The model under review builds one solid part; all positions refer to its coordinate system, in mm. A direction names the side the tool comes from. Coordinates: 2 decimals unless noted, no trailing zeros. Order: outer loops, then holes, each group sorted by start corner. A loop starts at its lowest first (then second) coordinate and runs counter-clockwise, first axis right, second up. Notation, with made-up numbers: M 34,42 L 80,42 A16 ccw 80,71 Z; hole C 23,-19.75 d2. An arc over 180 degrees is marked long. Write each question's results on one line, items separated by ' | '.
from build123d import *

# Parameters (mm, degrees)
SKETCH1_W                    = 168.275
SKETCH1_H                    = 76.2
EXTRUDE1_DEPTH               = 57.15
SKETCH2_R                    = 12.7
EXTRUDE2_DEPTH               = 6.35
SKETCH3_R                    = 9.525
EXTRUDE3_DEPTH               = 38.1
F_5_16_18_TAPPED_HOLE1_D     = 6.5278
F_5_16_18_TAPPED_HOLE1_DEPTH = 22.9235
F_5_16_18_TAPPED_HOLE1_TIP   = 1.961148974
SKETCH7_R                    = 36.83
EXTRUDE4_DEPTH               = 68.072
SKETCH8_R                    = 38.481
EXTRUDE5_DEPTH               = 25.4
F_5_16_18_TAPPED_HOLE2_D     = 6.5278
F_5_16_18_TAPPED_HOLE2_DEPTH = 22.922992
F_5_16_18_TAPPED_HOLE2_TIP   = 1.961148974
SKETCH11_OUTSIDE_W           = 224.478
SKETCH11_OUTSIDE_H           = 132.784
CUT_EXTRUDE1_DEPTH           = 9.525


with BuildPart() as part:
    # Sketch1 → Extrude1 (new body)
    with BuildSketch(Plane.XY):
        with Locations((41.7703, 0)):
            Rectangle(SKETCH1_W, SKETCH1_H)
    extrude(amount=-EXTRUDE1_DEPTH)

    # Sketch2 → Extrude2 (add)
    with BuildSketch(Plane.XY):
        Circle(SKETCH2_R)
    extrude(amount=EXTRUDE2_DEPTH)

    # Sketch3 → Extrude3 (add)
    with BuildSketch(Plane.XY.offset(6.35)):
        Circle(SKETCH3_R)
    extrude(amount=EXTRUDE3_DEPTH)

    # 5/16-18 Tapped Hole1
    with Locations(Plane.XZ.offset(38.1)):
        with Locations((-34.4297, -23.8125), (-34.4297, -49.2125), (117.9703, -49.2125), (117.9703, -23.8125)):
            Hole(F_5_16_18_TAPPED_HOLE1_D / 2, depth=F_5_16_18_TAPPED_HOLE1_DEPTH)
            with Locations((0, 0, -(F_5_16_18_TAPPED_HOLE1_DEPTH + F_5_16_18_TAPPED_HOLE1_TIP / 2))):  # 118° drill point
                Cone(0, F_5_16_18_TAPPED_HOLE1_D / 2, F_5_16_18_TAPPED_HOLE1_TIP, mode=Mode.SUBTRACT)

    # Sketch7 → Extrude4 (add)
    with BuildSketch(Plane(origin=(0, 0, -57.15), x_dir=(-1, 0, 0), z_dir=(0, 0, -1))):
        with Locations((-87.8078, 0)):
            Circle(SKETCH7_R)
    extrude(amount=EXTRUDE4_DEPTH)

    # Sketch8 → Extrude5 (add)
    with BuildSketch(Plane(origin=(0, 0, -125.222), x_dir=(-1, 0, 0), z_dir=(0, 0, -1))):
        with Locations((-87.8078, 0)):
            Circle(SKETCH8_R)
    extrude(amount=EXTRUDE5_DEPTH)

    # 5/16-18 Tapped Hole2
    with Locations(Plane(origin=(0, 38.1, 0), x_dir=(-1, 0, 0), z_dir=(0, 1, 0))):
        with Locations((34.4297, -23.8125), (34.4297, -49.2125), (-117.9703, -49.2125), (-117.9703, -23.8125)):
            Hole(F_5_16_18_TAPPED_HOLE2_D / 2, depth=F_5_16_18_TAPPED_HOLE2_DEPTH)
            with Locations((0, 0, -(F_5_16_18_TAPPED_HOLE2_DEPTH + F_5_16_18_TAPPED_HOLE2_TIP / 2))):  # 118° drill point
                Cone(0, F_5_16_18_TAPPED_HOLE2_D / 2, F_5_16_18_TAPPED_HOLE2_TIP, mode=Mode.SUBTRACT)

    # Sketch11 outside → Cut-Extrude1 (cut)
    with BuildSketch(Plane.XY):
        with Locations((41.961, 0)):
            Rectangle(SKETCH11_OUTSIDE_W, SKETCH11_OUTSIDE_H)
        with BuildLine():
            Line((89.393090644, 18.410189037), (27.411408932, 18.410189037))
            ThreePointArc((27.411408932, 18.410189037), (-33.006603821, 0.940480831), (26.318636507, -19.941157749))
            Line((26.318636507, -19.941157749), (89.393090644, -19.941157749))
            ThreePointArc((89.393090644, -19.941157749), (108.568764037, -0.765484356), (89.393090644, 18.410189037))
        make_face(mode=Mode.SUBTRACT)
    extrude(amount=-CUT_EXTRUDE1_DEPTH, mode=Mode.SUBTRACT)


solid = part.part
1) For pin 1 (8 mm diameter, centred on y = -9.5, z = -21.5, fed in from +X); pin 2 (8.5 mm diameter, centred on x = 117.97, z = -49.21, fed in from +Y); pin 3 (7.5 mm diameter, centred on x = 62.5, z = -3, fed in from +Y), all flat-tipped, find the tip position at first contact; note any pin that passes through.
Solutions:
pin 1: x = 125.91 | pin 2: y = 38.1 | pin 3: y = 18.41
2) Take a section at A-A on x = 0. State the section outline as (y, z) points (3 decimals), plus the area to 3 significant figures.
Solutions:
outline: M -38.1,-57.15 L 38.1,-57.15 L 38.1,-9.525 L 33.02,-9.525 L 33.02,0 L 12.7,0 L 12.7,6.35 L 9.525,6.35 L 9.525,44.45 L -9.525,44.45 L -9.525,6.35 L -12.7,6.35 L -12.7,0 L -33.02,0 L -33.02,-9.525 L -38.1,-9.525 Z | area: 5,150 mm2
3) Take a section at C-C on y = 0. State the section outline as (x, z) points (3 decimals), plus the area to 3 significant figures.
Solutions:
outline: M -42.367,-57.15 L 50.978,-57.15 L 50.978,-125.222 L 49.327,-125.222 L 49.327,-150.622 L 126.289,-150.622 L 126.289,-125.222 L 124.638,-125.222 L 124.638,-57.15 L 125.908,-57.15 L 125.908,-9.525 L 108.553,-9.525 L 108.553,0 L 12.7,0 L 12.7,6.35 L 9.525,6.35 L 9.525,44.45 L -9.525,44.45 L -9.525,6.35 L -12.7,6.35 L -12.7,0 L -33.02,0 L -33.02,-9.525 L -42.367,-9.525 Z | area: 17,200 mm2
4) Take a section at D-D on x = 43. State the section outline as (y, z) points (3 decimals), plus the area to 3 significant figures.
Solutions:
outline: M -38.1,-57.15 L 38.1,-57.15 L 38.1,-9.525 L 18.41,-9.525 L 18.41,0 L -19.941,0 L -19.941,-9.525 L -38.1,-9.525 Z | area: 3,990 mm2
5) To check wall thickness, follow line 1 along Z through (x, y) = (60, -14); line 2 along Z through (x, y) = (71, -20) (3 decimals); line 3 along Y through (x, z) = (56, -32). State the ranges of each line that lie inside material, in increasing order.
Solutions:
line 1: -150.62 to 0 | line 2: -150.622 to -9.525 | line 3: -38.1 to 38.1
6) Take a section at B-B on z = -65.5. State the section outline as (x, y) points.
Solutions:
outline: C 87.81,0 d73.66
7) For faces 1 (the cylindrical face through (-2.75, -12.4, 3.13)), 2 (the cylindrical face through (-36.184, -26.478, -46.46)), 3 (the flat face through (88, -37, -125.222)), list the 3-axis set-ups (+Z, -Z, +X, -X, +Y, -Y) from which the entire face can be reached by the end or side of a thin tool; tool diameter is ignored.
Solutions:
face 1: +Z | face 2: -Y | face 3: none
8) The part is to be moulded in two halves that separate along X. For faces 4 (the cylindrical face through (124.602, 1.619, -90.709)), 5 (the flat face through (0, 0, 44.45)), 6 (the conical face through (118.388, 13.556, -23.429)), say which applies: pulls with the +X half, pulls with the -X half, needs draft (parallel to the pull), parting line crosses it, or undercut.
Solutions:
face 4: parting line crosses it | face 5: needs draft | face 6: undercut
